```python
from build123d import *

# Parameters (mm, degrees)
SKETCH1_W           = 6
SKETCH1_H           = 6
BOSS_EXTRUDE1_DEPTH = 5
CUT_EXTRUDE1_DEPTH  = 10
CUT_EXTRUDE2_DEPTH  = 3
CUT_EXTRUDE3_DEPTH  = 3


with BuildPart() as part:
    # Sketch1 → Boss-Extrude1 (new body)
    with BuildSketch(Plane(origin=(0, 0, 0), x_dir=(1, 0, 0), z_dir=(0, 1, 0))):
        Rectangle(SKETCH1_W, SKETCH1_H)
    extrude(amount=BOSS_EXTRUDE1_DEPTH)

    # Sketch2 → Cut-Extrude1 (cut)
    with BuildSketch(Plane.ZY.offset(3)):
        Polygon((3, 5), (-3, 5), (0, 2.5), align=None)
    extrude(amount=-CUT_EXTRUDE1_DEPTH, mode=Mode.SUBTRACT)

    # Sketch3 → Cut-Extrude2 (cut)
    with BuildSketch(Plane(origin=(3, 0, 0), x_dir=(0, 0, -1), z_dir=(1, 0, 0))):
        Polygon((-3, 0), (0, 2.5), (-3, 5), align=None)
    extrude(amount=-CUT_EXTRUDE2_DEPTH, mode=Mode.SUBTRACT)

    # Sketch4 → Cut-Extrude3 (cut)
    with BuildSketch(Plane.ZY.offset(3)):
        Polygon((0, 0), (3, 0), (3, 2), align=None)
    extrude(amount=-CUT_EXTRUDE3_DEPTH, mode=Mode.SUBTRACT)


solid = part.part
```
Part model, mm, in its own coordinate system. A direction names the side the tool comes from. Round coordinates to 2 decimals unless told otherwise and drop trailing zeros. Loops run counter-clockwise (first coordinate to the right, second up) from the corner with the lowest first, then second, coordinate; pieces in that order, holes last.
1. Slice it at A-A (y = 3.15). Give the cut face in (x, z), and give its area (3 significant figures).
Solutions:
outline: (-3, -3) - (3, -3) - (3, -0.78) - (-3, -0.78) - close; (-3, 0.78) - (0, 0.78) - (0, 3) - (-3, 3) - close
area: 20.0 mm2
2. Drill centre lines: line 1 along X through (y, z) = (3.5, 1.85); line 2 along Z through (x, y) = (-2.35, 2.6); line 3 along Z through (x, y) = (-0.05, 4.65). Where is each one in solid material? Low to high.
Solutions:
line 1: x = -3 to 0
line 2: z = -3 to -0.12, 0.12 to 3
line 3: z = -3 to -2.58, 2.58 to 3
3. Slice it at C-C (x = -2.15). Give the cut face in (y, z).
Solutions:
outline: (0, -3) - (5, -3) - (2.5, 0) - (5, 3) - (2, 3) - (0, 0) - close
4. Slice it at D-D (z = 0.9). Give the cut face in (x, y).
Solutions:
outline: (-3, 0.6) - (0, 0.6) - (0, 0) - (3, 0) - (3, 1.75) - (0, 1.75) - (0, 3.25) - (-3, 3.25) - close
5. Slice it at B-B (z = 2.55). Give the cut face in (x, y) (3 decimals).
Solutions:
outline: (-3, 1.7) - (0, 1.7) - (0, 4.625) - (-3, 4.625) - close; (0, 0) - (3, 0) - (3, 0.375) - (0, 0.375) - close
6. 3-axis set-ups, long thin cutter, end or side, ignore diameter. For faces 1 (the face through (-3, 2, 0)), 2 (the face through (-1.5, 1, 1.5)), 3 (the face through (0, 3, 2)): which of +Z, -Z, +X, -X, +Y, -Y reach the whole face in a straight line?
Solutions:
face 1: +Z, -Z, -X, +Y, -Y
face 2: +Z, -X, -Y
face 3: +Z, +X, +Y
7. Flat gauge pins, fed straight in: pin 1 (1.5 mm diameter, centred on x = 1, z = -1, fed in from +Y); pin 2 (3 mm diameter, centred on x = 2, y = 2.5, fed in from +Z). Where does each tip first touch, or does it go through?
Solutions:
pin 1: stops at y = 3.96
pin 2: stops at z = 1.8
8. Two-plate mould, pull along Z, no slides. Class faces 4 (the face through (0, 2, -3)), 5 (the face through (0.62, 3.09, -0.71)), 6 (the face through (-1.521, 3.732, 1.479)), 7 (the face through (0, 0.3, 1.5)): pulls with the +Z half, pulls with the -Z half, needs draft (parallel to the pull), parting line crosses it, or undercut.
Solutions:
face 4: pulls with the -Z half
face 5: undercut
face 6: undercut
face 7: needs draft
